For this review, take the finished solid that the model builds, in its own axes (mm). A direction names the side the tool comes from. Round coordinates to 2 decimals unless told otherwise and drop trailing zeros. Order: outer loops, then holes, each group sorted by start corner. A loop starts at its lowest first (then second) coordinate and runs counter-clockwise, first axis right, second up.
Autodesk Inventor part; units mm, degrees
ref_plane "YZ Plane" through (0, 0, 0) normal (1, 0, 0) x (0, 1, 0)
ref_plane "XZ Plane" through (0, 0, 0) normal (0, 1, 0) x (-1, 0, 0)
ref_plane "XY Plane" through (0, 0, 0) normal (0, 0, 1) x (1, 0, 0)
sketch "Sketch1" plane through (0, 0, 0) normal (0, 0, 1) x (1, 0, 0)
  line L0 (0, 0) -> (25, 0)
  line L1 (25, 0) -> (25, 40)
  line L2 (25, 40) -> (0, 40)
  line L3 (0, 40) -> (0, 0)
  dimension "d1" = 25
  dimension "d2" = 40
  dimension "d3" = 25
extrude "Extrusion1" add sketch "Sketch1" against normal blind 30
sketch "Sketch2" plane through (25, 0, 0) normal (1, 0, 0) x (0, 0, -1)
  line L0 (0, 0) -> (30, 0)
  circle A0 centre (15, 6.56) radius 2.46
extrude "Extrusion2" cut sketch "Sketch2" against normal blind 30
sketch "Sketch3" plane through (0, 0, 0) normal (-1, 0, 0) x (0, 0, 1)
  line L0 (0, 0) -> (-30, 0)
  line L1 (-25.05, 0) -> (-4.95, 0)
  line L2 (-4.95, 0) -> (-4.95, 33.12)
  line L3 (-4.95, 33.12) -> (-25.05, 33.12)
  line L4 (-25.05, 33.12) -> (-25.05, 0)
  dimension "d11" = 20.1
extrude "Extrusion3" cut sketch "Sketch3" against normal blind 20
sketch "Sketch4" plane through (0, 0, 0) normal (0, -1, 0) x (1, 0, 0)
  line L0 (20, -4.95) -> (20, -25.05)
  line L1 (20, -15) -> (25, -15)
  line L2 (25, 0) -> (25, -30)
  line L3 (20, -8.025) -> (25, -8.025)
  line L4 (25, -8.025) -> (25, -21.975)
  line L5 (25, -21.975) -> (20, -21.975)
  line L6 (20, -21.975) -> (20, -8.025)
  line L7 (20, -8.025) -> (25, -21.975) construction
  line L8 (25, -8.025) -> (20, -21.975) construction
  line L9 (25, -12.54) -> (25, -17.46)
  point P0 (0, 0)
  point P1 (22.5, -15)
  dimension "d14" = 13.95
extrude "Extrusion4" add sketch "Sketch4" along normal blind 15
sketch "Sketch5" plane through (20, 0, 0) normal (-1, 0, 0) x (0, 0, 1)
  circle A0 centre (-15, 6.56) radius 2.46
  circle A1 centre (-15, 6.56) radius 4.7025
  circle A2 centre (-15, 6.56) radius 2.46
  circle A3 centre (-15, 6.56) radius 2.46
  point P0 (0, 0)
  dimension "d17" = 9.405
extrude "Extrusion5" cut sketch "Sketch5" against normal blind 2.1
sketch "Sketch6" plane through (25, 0, 0) normal (1, 0, 0) x (0, 0, -1)
  circle A0 centre (15, 6.56) radius 4.7025
  line L0 (15, 6.56) -> (15, 23.56)
  circle A1 centre (15, 23.56) radius 2.46
  point P0 (0, 0)
  dimension "d20" = 17
  dimension "d21" = 4.92
extrude "Extrusion6" cut sketch "Sketch6" against normal blind 10 contours A1
sketch "Sketch7" plane through (20, 0, 0) normal (-1, 0, 0) x (0, 0, 1)
  circle A0 centre (-15, 23.56) radius 2.46
  circle A1 centre (-15, 23.56) radius 4.7025
  point P0 (0, 0)
  dimension "d24" = 9.405
extrude "Extrusion7" cut sketch "Sketch7" against normal blind 2.1
sketch "Sketch9" plane through (25, 0, 0) normal (1, 0, 0) x (0, 0, -1)
  circle A0 centre (15, 6.56) radius 2.46
  circle A1 centre (15, 6.56) radius 2.46
  circle A2 centre (15, 23.56) radius 2.46
  circle A3 centre (15, 23.56) radius 2.46
  line L0 (30, 40) -> (30, 0)
  line L1 (30, 0) -> (30, 40)
  line L2 (30, 40) -> (0, 40)
  line L3 (0, 40) -> (0, 0)
  line L4 (0, 0) -> (8.025, 0)
  line L5 (21.975, 0) -> (21.975, -15)
  line L6 (21.975, -15) -> (8.025, -15)
  line L7 (8.025, -15) -> (8.025, 0)
  line L8 (0, 0) -> (8.025, 0)
  line L9 (21.975, 0) -> (30, 0)
extrude "Extrusion8" add sketch "Sketch9" along normal blind 5
sketch "Sketch10" plane through (0, 40, 0) normal (0, 1, 0) x (1, 0, 0)
  line L0 (0, 30) -> (30, 30)
  line L1 (30, 0) -> (0, 0)
  line L2 (0, 30) -> (30, 30)
  line L3 (30, 30) -> (30, 0)
  line L4 (30, 0) -> (0, 0)
  line L5 (0, 0) -> (0, 30)
extrude "Extrusion9" add sketch "Sketch10" along normal blind 15
sketch "Sketch12" plane through (30, 0, 0) normal (1, 0, 0) x (0, 0, -1)
  circle A0 centre (15, 6.56) radius 2.46
  line L0 (15, 6.56) -> (15, 15.06)
  circle A1 centre (15, 15.06) radius 2.525
  point P0 (0, 0)
  dimension "d31" = 8.5
  dimension "d33" = 5.05
extrude "Extrusion10" cut sketch "Sketch12" against normal blind 30 contours A1
sketch "Sketch15" plane through (0, 0, -25.05) normal (-1, 0, 0) x (0, 0, 1)
  line L0 (0, 33.12) -> (20.1, 33.12)
  line L1 (20.1, 33.12) -> (20.1, 0)
  line L2 (0, 33.12) -> (20.1, 33.12)
  line L3 (20.1, 33.12) -> (20.1, 31.1)
  line L4 (20.1, 31.1) -> (0, 31.1)
  line L5 (0, 31.1) -> (0, 33.12)
  point P0 (25.05, 0)
  dimension "d57" = 2.02
extrude "Extrusion13" add sketch "Sketch15" against normal blind 20
sketch "Sketch17" plane through (0, 0, 0) normal (0, 0, 1) x (1, 0, 0)
  line L0 (0, 55) -> (30, 55)
  line L1 (0, 55) -> (0, 0)
  line L2 (0, 55) -> (30, 55)
  line L3 (4, 73) -> (0, 75)
  line L4 (4, 57) -> (0, 55)
  line L5 (4, 57) -> (8, 65)
  line L6 (4, 73) -> (8, 65)
  line L7 (0, 75) -> (30, 75)
  line L8 (30, 55) -> (30, 75)
extrude "Extrusion14" add sketch "Sketch17" against normal blind 30
sketch "Sketch23" plane through (30, 0, 0) normal (1, 0, 0) x (0, 0, -1)
  circle A0 centre (15, 6.56) radius 2.46
  circle A1 centre (15, 6.56) radius 3.5
  circle A2 centre (15, 23.56) radius 2.46
  circle A3 centre (15, 23.56) radius 3.5
  point P0 (0, 0)
  dimension "d88" = 7
  dimension "d89" = 7
extrude "Extrusion16" cut sketch "Sketch23" against normal blind 10
properties part number "rec_c_16mm_x_120mm"
Q1. Take a section at C-C, the plane z = -15. Count the separate pieces of the cut face and the enclosed holes in it, plus the area to 3 significant figures.
Q2. Take a section at D-D, the plane x = 28.25. State the section outline as (y, z) points (3 decimals), plus the area to 3 significant figures.
Q3. Wall thickness on line 1 (Y direction, x = 27.75, z = -15) (3 decimals); line 2 (Y direction, x = 21.2, z = -15) (1 decimal); line 3 (Z direction, x = 26.75, y = 15.06) (3 decimals): over which ranges is each line inside the solid? List them lowest first.
Q4. Take a section at B-B, the plane y = 15.06. State the section outline as (x, z) points (3 decimals).
Q5. Take a section at A-A, the plane x = 6.5. State the section outline as (y, z) points, plus the area to 3 significant figures.
Q6. Tool access review of faces 1 (the face through (25, -8, -8.025)), 2 (the face through (22.1, 6, -19)), 3 (the face through (10, 31.1, -15)), 4 (the face through (25, -7, -21.975)): name each direction out of +Z, -Z, +X, -X, +Y, -Y from which nothing blocks a thin tool from reaching the whole face with its end or side.
Q7. Mouldability with a two-part tool opening along Z and no side actions: class faces 5 (the face through (15, 38, 0)), 6 (the face through (21.035, 7.973, -10.515)), 7 (the face through (6, 69, -15)) as +Z half, -Z half, draft (parallel to the pull), parting line (faces both ways), or undercut.
Q8. Clearance check with flat-ended pins moving along their axes: pin 1 (9 mm diameter, centred on x = 19, z = -26.5, fed in from -Y); pin 2 (6 mm diameter, centred on y = 3, z = -13, fed in from -X); pin 3 (3 mm diameter, centred on y = 6, z = -13.5, fed in from -X); pin 4 (8 mm diameter, centred on x = 4.5, z = -10, fed in from -Y). State where each tip first meets the part, or that it passes through.
Working result:
1. separate pieces: 4
1. enclosed holes: 0
1. area: 1,470 mm2
2. outline: (-15, -21.975) - (0, -21.975) - (0, -30) - (75, -30) - (75, 0) - (0, 0) - (0, -8.025) - (-15, -8.025) - close; hole circle Ø7 at (6.56, -15); hole circle Ø5.05 at (15.06, -15); hole circle Ø7 at (23.56, -15)
2. area: 2,360 mm2
3. line 1: y = -15 to 3.06, 10.06 to 12.535, 17.585 to 20.06, 27.06 to 75
3. line 2: y = -15 to 1.9, 11.3 to 12.5, 17.6 to 18.9, 28.3 to 75
3. line 3: z = -30 to -17.525, -12.475 to 0
4. outline: (0, -30) - (30, -30) - (30, -17.525) - (20, -17.525) - (20, -25.05) - (0, -25.05) - close; (0, -4.95) - (20, -4.95) - (20, -12.475) - (30, -12.475) - (30, 0) - (0, 0) - close
5. outline: (0, -30) - (62, -30) - (62, 0) - (0, 0) - (0, -4.95) - (31.1, -4.95) - (31.1, -25.05) - (0, -25.05) - close; (68, -30) - (75, -30) - (75, 0) - (68, 0) - close
5. area: 1,440 mm2
6. face 1: +Z, +X, -X, -Y
6. face 2: -X
6. face 3: -X, -Y
6. face 4: -Z, +X, -X, -Y
7. face 5: +Z half
7. face 6: undercut
7. face 7: draft
8. pin 1: stops at y = 0
8. pin 2: stops at x = 20
8. pin 3: passes through
8. pin 4: stops at y = 31.1
